Part model, mm, in its own coordinate system. Face numbers are marked on the shaded views. A direction names the side the tool comes from. Coordinates: 2 decimals unless noted, no trailing zeros. Use a Markdown table: item, result. Add a question column.
1) Probe probe 1 along Y at (x, z) = (1.25, 3); probe 2 along Z at (x, y) = (1.5, 2.25); probe 3 along X at (y, z) = (2.5, 0.25). List the from-to ranges inside material, lowest first. Write a range as [from, to].
2) Drop a flat-ended pin along its axis: P1, Ø1.5, axis at x = 1, y = 4, coming from the +Z side. Give the stop position or say it passes through.
3) Tool access for the marked faces 1 and 2: list every direction of +Z, -Z, +X, -X, +Y, -Y with a clear straight run to the whole face (end or side of a thin tool).
from build123d import *

# Parameters (mm, degrees)
BOSS_EXTRUDE1_DEPTH = 4


with BuildPart() as part:
    # Sketch1 → Loft1 section 0
    with BuildSketch(Plane(origin=(0, 0, 0), x_dir=(1, 0, 0), z_dir=(0, 1, 0))):
        with BuildLine():
            Line((2.482606158, 0), (1.241303079, 2.15))
            Line((1.241303079, 2.15), (-1.241303079, 2.15))
            Line((-1.241303079, 2.15), (-2.482606158, 0))
            Line((-2.482606158, 0), (-1.241303079, -2.15))
            Line((-1.241303079, -2.15), (1.241303079, -2.15))
            Line((1.241303079, -2.15), (2.482606158, 0))
        make_face()
    # Sketch2 → Loft1 section 1
    with BuildSketch(Plane(origin=(0, 3, 0), x_dir=(1, 0, 0), z_dir=(0, 1, 0))):
        with BuildLine():
            Line((2.655811238, 0), (1.327905619, 2.3))
            Line((1.327905619, 2.3), (-1.327905619, 2.3))
            Line((-1.327905619, 2.3), (-2.655811238, 0))
            Line((-2.655811238, 0), (-1.327905619, -2.3))
            Line((-1.327905619, -2.3), (1.327905619, -2.3))
            Line((1.327905619, -2.3), (2.655811238, 0))
        make_face()
    loft()

    # Sketch3 → Boss-Extrude1 (add)
    with BuildSketch(Plane(origin=(0, 3, 0), x_dir=(1, 0, 0), z_dir=(0, 1, 0))):
        Polygon((0, 3.5), (0, 3.85), (0.607768622, 3.446827136), (0.668545484, 3.791509849), (1.197070502, 3.288924173), (1.316777552, 3.61781659), (1.75, 3.031088913), (1.925, 3.334197805), (2.249756634, 2.681155551), (2.474732297, 2.949271106), (2.681155551, 2.249756634), (2.949271106, 2.474732297), (3.031088913, 1.75), (3.334197805, 1.925), (3.288924173, 1.197070502), (3.61781659, 1.316777552), (3.446827136, 0.607768622), (3.791509849, 0.668545484), (3.5, 0), (3.85, 0), (3.446827136, -0.607768622), (3.791509849, -0.668545484), (3.288924173, -1.197070502), (3.61781659, -1.316777552), (3.031088913, -1.75), (3.334197805, -1.925), (2.681155551, -2.249756634), (2.949271106, -2.474732297), (2.249756634, -2.681155551), (2.474732297, -2.949271106), (1.75, -3.031088913), (1.925, -3.334197805), (1.197070502, -3.288924173), (1.316777552, -3.61781659), (0.607768622, -3.446827136), (0.668545484, -3.791509849), (0, -3.5), (0, -3.85), (-0.607768622, -3.446827136), (-0.668545484, -3.791509849), (-1.197070502, -3.288924173), (-1.316777552, -3.61781659), (-1.75, -3.031088913), (-1.925, -3.334197805), (-2.249756634, -2.681155551), (-2.474732297, -2.949271106), (-2.681155551, -2.249756634), (-2.949271106, -2.474732297), (-3.031088913, -1.75), (-3.334197805, -1.925), (-3.288924173, -1.197070502), (-3.61781659, -1.316777552), (-3.446827136, -0.607768622), (-3.791509849, -0.668545484), (-3.5, 0), (-3.85, 0), (-3.446827136, 0.607768622), (-3.791509849, 0.668545484), (-3.288924173, 1.197070502), (-3.61781659, 1.316777552), (-3.031088913, 1.75), (-3.334197805, 1.925), (-2.681155551, 2.249756634), (-2.949271106, 2.474732297), (-2.249756634, 2.681155551), (-2.474732297, 2.949271106), (-1.75, 3.031088913), (-1.925, 3.334197805), (-1.197070502, 3.288924173), (-1.316777552, 3.61781659), (-0.607768622, 3.446827136), (-0.668545484, 3.791509849), align=None)
    extrude(amount=BOSS_EXTRUDE1_DEPTH)


solid = part.part
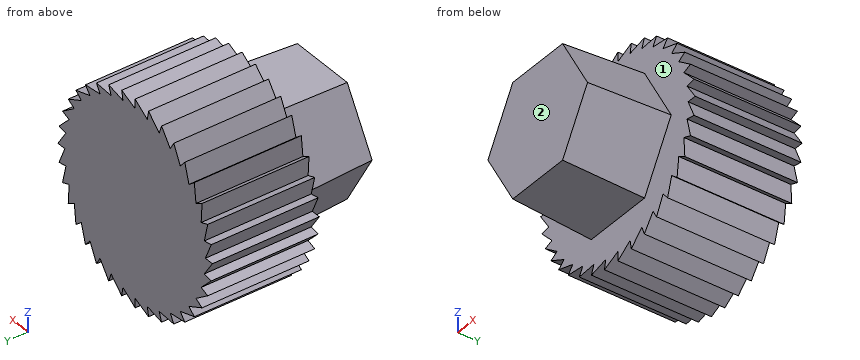
Answer block:
| question | item | result |
|---|---|---|
| 1 | probe 1 | [3, 7] |
| 1 | probe 2 | [-1.93, 1.93] |
| 1 | probe 3 | [-2.48, 2.48] |
| 2 | P1 | z = 3.79 |
| 3 | face 1 | -Y |
| 3 | face 2 | +Z, -Z, +X, -X, -Y |
